The drawing under review shows one solid part. Ordinate dimensions are in mm from its lowest x, y, z. A direction names the side the tool comes from. Coordinates: 2 decimals unless noted, no trailing zeros. Loops run counter-clockwise (first coordinate to the right, second up) from the corner with the lowest first, then second, coordinate; pieces in that order, holes last. Notation, with made-up numbers: M 75.5,87 L 134.5,87 A29 ccw 134.5,125 Z; hole C 40,-28.75 d9. An arc over 180 degrees is marked long. Use one line per item in the form item = value.
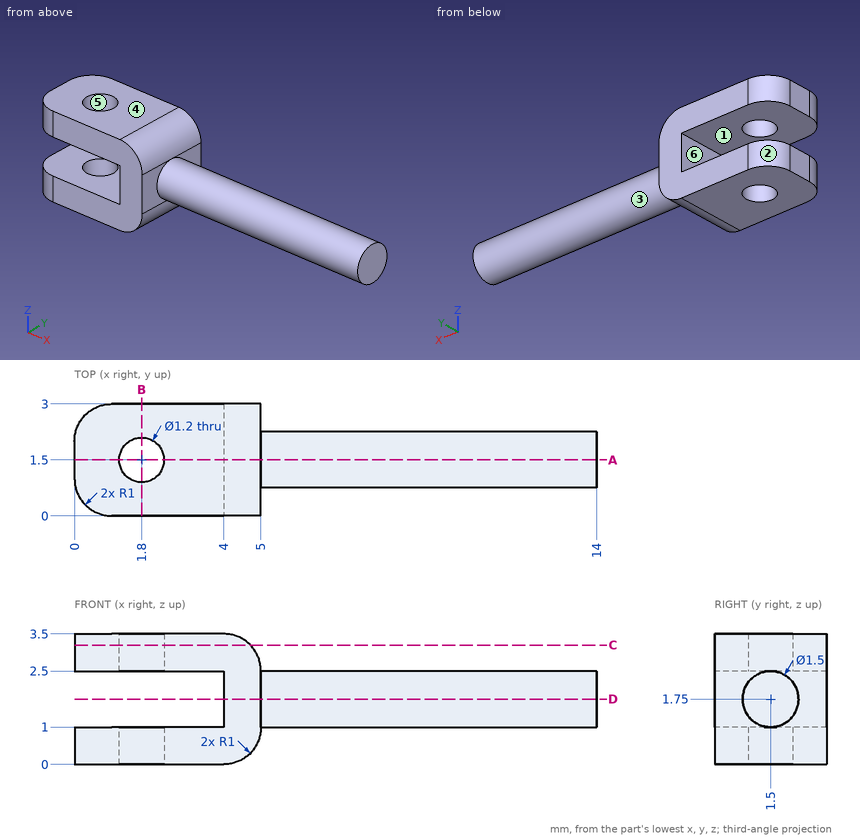
1. Consider section C-C on z = 3.2. Write out the cut boundary in (x, y), plus the area to 3 significant figures.
Computed values:
outline = M 0,1 A1 ccw 1,0 L 4.71,0 L 4.71,3 L 1,3 A1 ccw 0,2 Z; hole C 1.8,1.5 d1.2
area = 12.6 mm2
2. For pin 1 Ø1.5 at (x, z) = (8.5, 1.5) entering from +Y, flat-tipped, find the tip position at first contact; note if it passes through.
Computed values:
pin_1 = 2.25
3. Wall thickness on line 1 along Y through (x, z) = (1.8, 3.2); line 2 along Z through (x, y) = (1.25, 1.9); line 3 along X through (y, z) = (1.45, 2.35): over which ranges is each line inside the solid? List them lowest first. Write a range as from..to.
Computed values:
line_1 = 0..0.9, 2.1..3
line_2 = 0..1, 2.5..3.5
line_3 = 4..14
4. Consider section D-D on z = 1.75. Write out the cut boundary in (x, y), plus the area to 3 significant figures.
Computed values:
outline = M 4,0 L 5,0 L 5,0.75 L 14,0.75 L 14,2.25 L 5,2.25 L 5,3 L 4,3 Z
area = 16.5 mm2
5. Consider section B-B on x = 1.8. Write out the cut boundary in (y, z).
Computed values:
outline = M 0,0 L 0.9,0 L 0.9,1 L 0,1 Z; M 0,2.5 L 0.9,2.5 L 0.9,3.5 L 0,3.5 Z; M 2.1,0 L 3,0 L 3,1 L 2.1,1 Z; M 2.1,2.5 L 3,2.5 L 3,3.5 L 2.1,3.5 Z
6. Tool access review of the marked faces 1, 2 and 3: name each direction out of +Z, -Z, +X, -X, +Y, -Y from which nothing blocks a thin tool from reaching the whole face with its end or side.
Computed values:
face_1 = -X, +Y, -Y
face_2 = +Z, -Z, -X, +Y
face_3 = +X
7. Consider section A-A on y = 1.5. State how many separate pieces and enclosed holes the cut face has, plus the area to 3 significant figures.
Computed values:
separate_pieces = 3
enclosed_holes = 0
area = 22.2 mm2
8. Draft analysis for pull direction Z (two halves, no side actions). For the marked faces 4, 5 and 6, state which applies: +Z half, -Z half, draft (parallel to the pull), parting line (faces both ways), or undercut.
Computed values:
face_4 = +Z half
face_5 = draft
face_6 = undercut
